Design review of the part built by this model. Coordinates are the model's own, in mm. Coordinates: 2 decimals unless noted, no trailing zeros. Write each loop counter-clockwise with the first axis right and the second up, starting at its lowest first coordinate (ties: lowest second). Pieces come first, ordered by that corner, then holes. Notation, with made-up numbers: M -4.75,-4 L 42.25,-4 A26 cw 42.25,11 Z; hole C 58,77.25 d5. An arc over 180 degrees is marked long. One line per question, with ' | ' between items.
Autodesk Inventor part; units mm, degrees
ref_plane "YZ Plane" through (0, 0, 0) normal (1, 0, 0) x (0, 1, 0)
ref_plane "XZ Plane" through (0, 0, 0) normal (0, 1, 0) x (-1, 0, 0)
ref_plane "XY Plane" through (0, 0, 0) normal (0, 0, 1) x (1, 0, 0)
sketch "Sketch1" plane through (0, 0, 0) normal (0, 1, 0) x (-1, 0, 0)
  line L0 (47.9603, 101.1149) -> (-52.1157, 101.1149)
  line L1 (-52.1157, 101.1149) -> (-52.1157, -254.4851)
  line L2 (-52.1157, -254.4851) -> (47.9603, -254.4851)
  line L3 (47.9603, -254.4851) -> (47.9603, 101.1149)
  point P0 (0, 0)
  dimension "d0" = 100.076
  dimension "d1" = 355.6
extrude "Extrusion1" add sketch "Sketch1" along normal blind 5.4102
sketch "Sketch5" plane through (0, 5.4102, 0) normal (0, 1, 0) x (1, 0, 0)
  circle A0 centre (-34.7523, 244.8585) radius 1.5
  circle A1 centre (38.9077, 244.8585) radius 1.5
  line L0 (-34.7355, 243.3586) -> (38.8909, 243.3586)
  line L1 (52.1157, 254.4851) -> (-47.9603, 254.4851)
  point P0 (0, 0)
  point P1 (2.0777, 243.3586)
  point P2 (2.0777, 254.4851)
  dimension "d8" = 3
  dimension "d9" = 3
  dimension "d10" = 73.66
  dimension "d11" = 9.6266
extrude "Extrusion3" cut sketch "Sketch5" against normal blind 25.4
sketch "Sketch6" plane through (0, 5.4102, 0) normal (0, 1, 0) x (1, 0, 0)
  line L0 (-47.9603, -101.1149) -> (52.1157, -101.1149)
  line L1 (-47.9603, -101.1149) -> (-41.6103, -101.1149)
  line L2 (-41.6103, -101.1149) -> (-41.6103, -98.3209)
  line L3 (-41.6103, -98.3209) -> (-47.9603, -98.3209)
  line L4 (-47.9603, -98.3209) -> (-47.9603, -101.1149)
  line L5 (52.1157, -101.1149) -> (45.7657, -101.1149)
  line L6 (45.7657, -101.1149) -> (45.7657, -98.3209)
  line L7 (45.7657, -98.3209) -> (52.1157, -98.3209)
  line L8 (52.1157, -98.3209) -> (52.1157, -101.1149)
  point P0 (0, 0)
  dimension "d14" = 2.794
  dimension "d15" = 6.35
  dimension "d16" = 6.35
extrude "Extrusion4" cut sketch "Sketch6" against normal blind 25.4
sketch "Sketch7" plane through (45.7657, 5.4102, 98.3209) normal (0, 0, 1) x (1, 0, 0)
  circle A0 centre (3.175, -2.7051) radius 1.5
  line L0 (0, 0) -> (6.35, 0)
  line L1 (6.35, 0) -> (6.35, -5.4102)
  circle A1 centre (-90.551, -2.7051) radius 1.5
  line L2 (-93.726, 0) -> (-87.376, 0)
  line L3 (-93.726, -5.4102) -> (-93.726, 0)
  point P0 (-45.7657, -5.4102)
  point P1 (3.175, 0)
  point P2 (6.35, -2.7051)
  point P3 (-90.551, 0)
  point P4 (-93.726, -2.7051)
  dimension "d19" = 3
  dimension "d20" = 3
extrude "Extrusion5" cut sketch "Sketch7" against normal blind 254
sketch "Sketch8" plane through (-41.6103, 0, 101.1149) normal (0, 0, 1) x (1, 0, 0)
  line L0 (0, 5.4102) -> (87.376, 5.4102)
  line L1 (0, 0) -> (87.376, 0)
  line L2 (0, 5.4102) -> (87.376, 5.4102)
  line L3 (87.376, 5.4102) -> (87.376, 0)
  line L4 (87.376, 0) -> (0, 0)
  line L5 (0, 0) -> (0, 5.4102)
  point P0 (41.6103, 0)
extrude "Extrusion6" add sketch "Sketch8" along normal blind 54.5338
sketch "Sketch9" plane through (-47.9603, 5.4102, 98.3209) normal (0, 0, 1) x (1, 0, 0)
  line L0 (6.35, 0) -> (6.35, -5.4102)
  line L1 (0, 0) -> (6.35, 0)
  line L2 (6.35, 0) -> (6.35, -5.4102)
  line L3 (6.35, -5.4102) -> (0, -5.4102)
  line L4 (0, -5.4102) -> (0, 0)
  line L5 (100.076, 0) -> (100.076, -5.4102)
  line L6 (100.076, -5.4102) -> (93.726, -5.4102)
  line L7 (100.076, 0) -> (93.726, 0)
  line L8 (93.726, 0) -> (93.726, -5.4102)
  line L9 (93.726, -5.4102) -> (100.076, -5.4102)
  line L10 (100.076, -5.4102) -> (100.076, 0)
  circle A0 centre (96.901, -2.7051) radius 1.5
  circle A1 centre (3.175, -2.7051) radius 1.5
  point P0 (47.9603, -5.4102)
extrude "Extrusion7" add sketch "Sketch9" along normal blind 54.5338
sketch "Sketch10" plane through (0, 5.4102, 0) normal (0, 1, 0) x (1, 0, 0)
  line L0 (-37.6261, -131.8997) -> (38.5739, -131.8997) construction
  line L1 (-37.6261, -106.4997) -> (38.5739, -106.4997) construction
  line L2 (-47.9603, 254.4851) -> (-47.9603, -152.8547) construction
  line L3 (52.1157, -152.8547) -> (52.1157, 254.4851) construction
  line L4 (45.7657, -155.6487) -> (-41.6103, -155.6487) construction
  line L5 (-37.6261, -114.1197) -> (-12.2261, -114.1197) construction
  line L6 (-12.2261, -114.1197) -> (-12.2261, -124.2797) construction
  line L7 (-12.2261, -124.2797) -> (-37.6261, -124.2797) construction
  line L8 (-37.6261, -131.8997) -> (-37.6261, -124.2797) construction
  line L9 (-37.6261, -114.1197) -> (-37.6261, -106.4997) construction
  line L10 (38.5739, -114.1197) -> (13.1739, -114.1197) construction
  line L11 (13.1739, -114.1197) -> (13.1739, -124.2797) construction
  line L12 (13.1739, -124.2797) -> (38.5739, -124.2797) construction
  line L13 (38.5739, -131.8997) -> (38.5739, -124.2797) construction
  line L14 (38.5739, -114.1197) -> (38.5739, -106.4997) construction
  circle A0 centre (34.7639, -110.3097) radius 1.5
  circle A1 centre (34.7639, -128.0897) radius 1.5
  circle A2 centre (-33.816, -127.9782) radius 1.5
  circle A3 centre (-33.816, -110.1982) radius 1.5
  point P0 (0, 0)
  point P1 (38.5739, -110.3097)
  dimension "d27" = 76.2
  dimension "d28" = 25.4
  dimension "d31" = 23.749
  dimension "d32" = 7.62
  dimension "d33" = 7.62
  dimension "d34" = 25.4
  dimension "d35" = 25.4
  dimension "d36" = 68.58
  dimension "d37" = 17.78
  dimension "d38" = 17.78
  dimension "d39" = 68.58
  dimension "d40" = 3
  dimension "d41" = 3
  dimension "d42" = 3
  dimension "d43" = 3
  dimension "d44" = 3.81
  dimension "d45" = 25.4
  dimension "d46" = 25.4
  dimension "d47" = 7.62
  dimension "d48" = 7.62
  dimension "d49" = 7.62
  dimension "d50" = 7.62
  dimension "d51" = 76.2
  dimension "d52" = 25.4
  dimension "d53" = 25.4
  dimension "d54" = 17.78
extrude "Extrusion8" cut sketch "Sketch10" against normal blind 54.5338
sketch "Sketch11" plane through (0, 5.4102, 0) normal (0, 1, 0) x (1, 0, 0)
  line L0 (-41.6103, -155.6487) -> (45.7657, -155.6487) construction
  line L1 (43.9115, -155.6487) -> (43.9115, -13.9421) construction
  line L2 (43.9115, -13.9421) -> (52.1157, -13.9421) construction
  line L3 (52.1157, -152.8547) -> (52.1157, 254.4851) construction
  circle A0 centre (43.9115, -13.9421) radius 1.0922
  circle A1 centre (-7.8029, -13.9421) radius 1.0922
  circle A2 centre (43.9115, 43.9953) radius 1.0928
  circle A3 centre (-7.8029, 43.9953) radius 1.0922
  point P0 (0, 0)
  dimension "d57" = 141.7066
  dimension "d58" = 8.2042
  dimension "d59" = 2.1844
  dimension "d60" = 2.1844
  dimension "d62" = 51.7144
  dimension "d63" = 57.9374
  dimension "d64" = 57.9374
extrude "Extrusion9" cut sketch "Sketch11" against normal blind 54.5338
sketch "Sketch12" plane through (0, 5.4102, 0) normal (0, 1, 0) x (1, 0, 0)
  circle A0 centre (43.4543, 73.8403) radius 1.5367
  line L0 (52.1157, -152.8547) -> (52.1157, 254.4851)
  line L1 (52.1157, -152.8547) -> (45.7657, -152.8547)
  line L2 (46.0959, 58.6257) -> (46.0959, 133.7589) construction
  line L3 (46.0959, 58.6257) -> (-7.3203, 58.6257) construction
  line L4 (46.0959, 133.7589) -> (44.0639, 133.7589) construction
  line L5 (44.0639, 133.7589) -> (44.0639, 136.7053) construction
  line L6 (44.0639, 136.7053) -> (6.6751, 136.7053) construction
  line L7 (6.6751, 136.7053) -> (6.6751, 133.7589) construction
  line L8 (6.6751, 133.7589) -> (-7.2949, 133.7589) construction
  line L9 (-7.3203, 58.6257) -> (-7.2949, 133.7589) construction
  circle A1 centre (38.5521, 134.0637) radius 1.5367
  circle A2 centre (10.6629, 134.0637) radius 1.5367
  point P0 (0, 0)
  dimension "d67" = 3.0734
  dimension "d68" = 8.6614
  dimension "d69" = 226.695
  dimension "d89" = 15.2146
  dimension "d90" = 2.6416
  dimension "d91" = 75.1332
  dimension "d92" = 53.4162
  dimension "d93" = 2.032
  dimension "d94" = 2.9464
  dimension "d95" = 37.3888
  dimension "d96" = 13.97
  dimension "d97" = 75.1332
  dimension "d98" = 3.0734
  dimension "d99" = 2.6416
  dimension "d100" = 3.0734
  dimension "d101" = 2.6416
  dimension "d102" = 27.8892
  dimension "d103" = 7.5438
  dimension "d104" = 60.4226
extrude "Extrusion10" cut sketch "Sketch12" against normal blind 25.4
sketch "Sketch13" plane through (0, 5.4102, 0) normal (0, 1, 0) x (1, 0, 0)
  line L0 (44.9886, 149.6605) -> (-23.5191, 149.6605)
  line L1 (-23.5191, 149.6605) -> (-23.5191, 169.3907)
  line L2 (-23.5191, 169.3907) -> (44.9886, 169.3907)
  line L3 (44.9886, 169.3907) -> (44.9886, 149.6605)
  point P0 (0, 0)
extrude "Extrusion11" cut sketch "Sketch13" against normal blind 25.4
sketch "Sketch14" plane through (0, 5.4102, 0) normal (0, 1, 0) x (1, 0, 0)
  line L0 (-39.2837, 182.0907) -> (45.1561, 182.0907) construction
  line L1 (45.1561, 182.0907) -> (45.1561, 192.9873) construction
  line L2 (45.1561, 192.9873) -> (-39.2837, 192.9873) construction
  line L3 (-39.2837, 192.9873) -> (-39.2837, 182.0907) construction
  line L4 (-23.5191, 169.3907) -> (44.9886, 169.3907) construction
  circle A0 centre (40.7951, 187.539) radius 2.2274
  circle A1 centre (-34.9227, 187.539) radius 2.2274
  line L5 (-47.9603, 254.4851) -> (-47.9603, -152.8547) construction
  line L6 (52.1157, -152.8547) -> (52.1157, 254.4851) construction
  point P0 (0, 0)
  dimension "d107" = 84.4398
  dimension "d108" = 10.8966
  dimension "d109" = 12.7
  dimension "d110" = 2.1336
  dimension "d111" = 2.1336
  dimension "d114" = 6.9596
extrude "Extrusion12" cut sketch "Sketch14" against normal blind 25.4
sketch "Sketch15" plane through (0, 5.4102, 0) normal (0, 1, 0) x (1, 0, 0)
  circle A0 centre (30.5257, -47.4955) radius 1.5
  line L0 (-47.9603, 254.4851) -> (-47.9603, -152.8547)
  line L1 (-41.6103, -152.8547) -> (-47.9603, -152.8547)
  line L2 (52.1157, -152.8547) -> (52.1157, 254.4851)
  circle A1 centre (-24.0589, 81.4603) radius 1.5
  point P0 (0, 0)
  dimension "d117" = 3
  dimension "d119" = 105.3592
  dimension "d120" = 21.59
  dimension "d121" = 3
  dimension "d122" = 23.9014
  dimension "d123" = 234.315
extrude "Extrusion13" cut sketch "Sketch15" against normal blind 25.4
equation "\"d9\" = d8"
equation "\"d20\" = d19"
equation "\"d60\" = d59"
equation "\"d111\" = d110"
equation "\"d121\" = d117"
properties part number "Control Board"
1. Take a section at A-A (z = -56.5). Write out the cut boundary in (x, y), then the cut area to 3 significant figures.
Answer sheet:
outline: M -47.96,0 L 52.12,0 L 52.12,5.41 L -47.96,5.41 Z; hole C -44.79,2.71 d3; hole C 48.94,2.71 d3 | area: 527 mm^2
2. To check wall thickness, follow line 1 along X through (y, z) = (2.85, -86.5); line 2 along X through (y, z) = (3.7, -35); line 3 along Z through (x, y) = (6.5, 0.9). State the ranges of each line that lie inside material, in increasing order. Write a range as [from, to].
Answer sheet:
line 1: [-47.96, -46.28], [-43.29, 47.45], [50.43, 52.12] | line 2: [-47.96, -45.91], [-43.66, 47.82], [50.06, 52.12] | line 3: [-254.49, -169.39], [-149.66, 155.65]
3. Insertion check: pin 1 Ø2.5 at (x, z) = (-24.06, -81.46) entering from +Y; pin 2 Ø2 at (y, z) = (3, 154) entering from -X; pin 3 Ø2.5 at (x, y) = (48.94, 2.71) entering from +Z; pin 4 Ø0.8 at (y, z) = (2.5, 153.5) entering from +X. Each pin has a flat end and moves straight along its axis. Give the tip position at first contact, or say it passes through.
Answer sheet:
pin 1: through | pin 2: x = -41.61 | pin 3: z = -155.68 | pin 4: x = 45.77
